Could you check a few things on this model? Use its own coordinates, in mm. Face numbers are marked on the shaded views. Give positions to 0.01 mm unless a question says otherwise; leave off trailing zeros. Order: outer loops, then holes, each group sorted by start corner. A loop starts at its lowest first (then second) coordinate and runs counter-clockwise, first axis right, second up. Notation, with made-up numbers: M 75.25,-21 L 132.25,-21 A19 ccw 132.25,8 Z; hole C 30.5,16.5 d4. An arc over 180 degrees is marked long. Return JSON: item names as keys, results as strings. Group by question number.
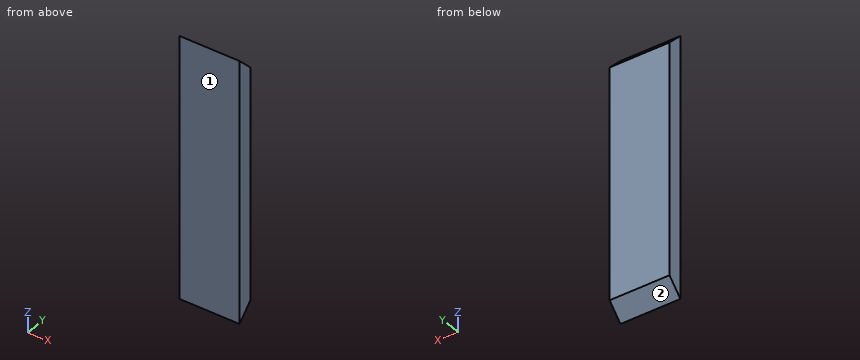
Autodesk Inventor part; units mm, degrees
ref_plane "Start plane" through (0, 0, 0) normal (0, 0, 1) x (1, 0, 0)
ref_plane "End plane" through (0, 0, 110.744) normal (0, 0, 1) x (1, 0, 0)
ref_plane "Work Plane4" through (0, -22.225, -19.05) normal (0, 0.7071, -0.7071) x (1, 0, 0)
ref_plane "Start plane" through (0, 0, 0) normal (0, 0, 1) x (1, 0, 0)
ref_plane "End plane" through (0, 0, 110.744) normal (0, 0, 1) x (1, 0, 0)
sketch "Sketch" plane through (0, 0, 0) normal (0, 0, 1) x (1, 0, 0)
  line L0 (12.7, -3.175) -> (-12.7, -3.175)
  line L1 (-12.7, -3.175) -> (-12.7, 3.175)
  line L2 (-12.7, 3.175) -> (12.7, 3.175)
  line L3 (12.7, 3.175) -> (12.7, -3.175)
  line L4 (-6, 0) -> (8, 0) construction
  line L5 (0, -30) -> (0, 40) construction
  line L6 (0, 54) -> (0, -44) construction
  line L7 (-17.78, 0) -> (17.78, 0) construction
  dimension "d0" = 6.35
  dimension "d1" = 25.4
  dimension "d4" = 12.7
  dimension "d5" = 3.175
extrude "Body" add sketch "Sketch" along normal up to surface (110.744 mm away) from surface at 0
sketch "Sketch3" plane through (0, 0, 0) normal (0, 0, 1) x (1, 0, 0)
  line L0 (0, 0) -> (10, 0)
ref_plane "Work Plane3" through (0, 0, 0) normal (0, -1, 0) x (1, 0, 0)
sketch "Sketch4" plane through (0, 0, 0) normal (0, -1, 0) x (1, 0, 0)
  line L0 (-2, 0) -> (12, 0)
  line L1 (-2, 110.744) -> (12, 110.744)
  dimension "d9" = 110.744
ref_plane "Work Plane4" through (0, -22.225, -19.05) normal (0, 0.7071, -0.7071) x (1, 0, 0)
split "Split1" plane through (0, -22.225, -19.05) removes the side toward (0, 0.7071, -0.7071)
ref_plane "Work Plane5" through (0, -3.175, 110.744) normal (0, 0.7071, 0.7071) x (1, 0, 0)
split "Split2" plane through (0, -3.175, 110.744) removes the side toward (0, 0.7071, 0.7071)
equation "\"d0\" = G_W"
equation "\"d1\" = G_H"
equation "\"d4\" = 0.5 * d1"
equation "\"d5\" = 0.5 * d0"
equation "\"d2\" = G_L"
equation "\"G_W\" = 6.35"
equation "\"G_H\" = 25.4"
equation "\"G_L\" = d9"
equation "\"G_OFFSET_START\" = 0"
equation "\"G_OFFSET_END\" = 0"
equation "\"d7\" = G_OFFSET_END + B_L"
equation "\"B_L\" = 110.744"
properties part number "AISC - 1/4x1 - 4.36" material "Steel, Mild"
1. If we mould it in two halves opening along Y, with no side actions, what happens to the marked faces 1 and 2? For each: pulls with the +Y half, pulls with the -Y half, needs draft (parallel to the pull), parting line crosses it, or undercut.
2. For pin 1 (1 mm diameter, centred on x = 2.5, y = -1.5, fed in from -Z) (3 decimals), with a flat end and sliding along its axis, tell me the tip position at first contact or that it passes through.
3. Imagine slicing it at A-A, the plane x = -7.25. Please give me the cut outline in (y, z) (3 decimals).
4. I need wall thicknesses on L1, parallel to Z at x = 8.25, y = 2 (3 decimals); L2, parallel to Z at x = 3, y = 0 (3 decimals). Which ranges of each line are inside material? Lowest first, please. Write a range as from..to.
5. Imagine slicing it at B-B, the plane y = 0. Please give me the cut outline in (x, z) (3 decimals), plus the area to 3 significant figures.
Values:
{
 "1": {"face 1": "pulls with the -Y half", "face 2": "pulls with the +Y half"},
 "2": {"pin 1": "stops at z = 1.175"},
 "3": {"outline": "M -3.175,0 L 3.175,6.35 L 3.175,104.394 L -3.175,110.744 Z"},
 "4": {"L1": "z = 5.175..105.569", "L2": "z = 3.175..107.569"},
 "5": {"outline": "M -12.7,3.175 L 12.7,3.175 L 12.7,107.569 L -12.7,107.569 Z", "area": "2,650 mm²"}
}
